Design review of the part shown in the three views and the two pictorial views. Dimensions are in mm from the part's minimum x, y and z. A direction names the side the tool comes from. Round coordinates to 2 decimals unless told otherwise and drop trailing zeros. Order: outer loops, then holes, each group sorted by start corner. A loop starts at its lowest first (then second) coordinate and runs counter-clockwise, first axis right, second up. Notation, with made-up numbers: (89.5, 13.5) - (133.5, 13.5) arc R9 cw to (133.5, 23.5) - close; hole circle Ø4 at (33, 74). An arc over 180 degrees is marked (long way). One line per item, written item: value.
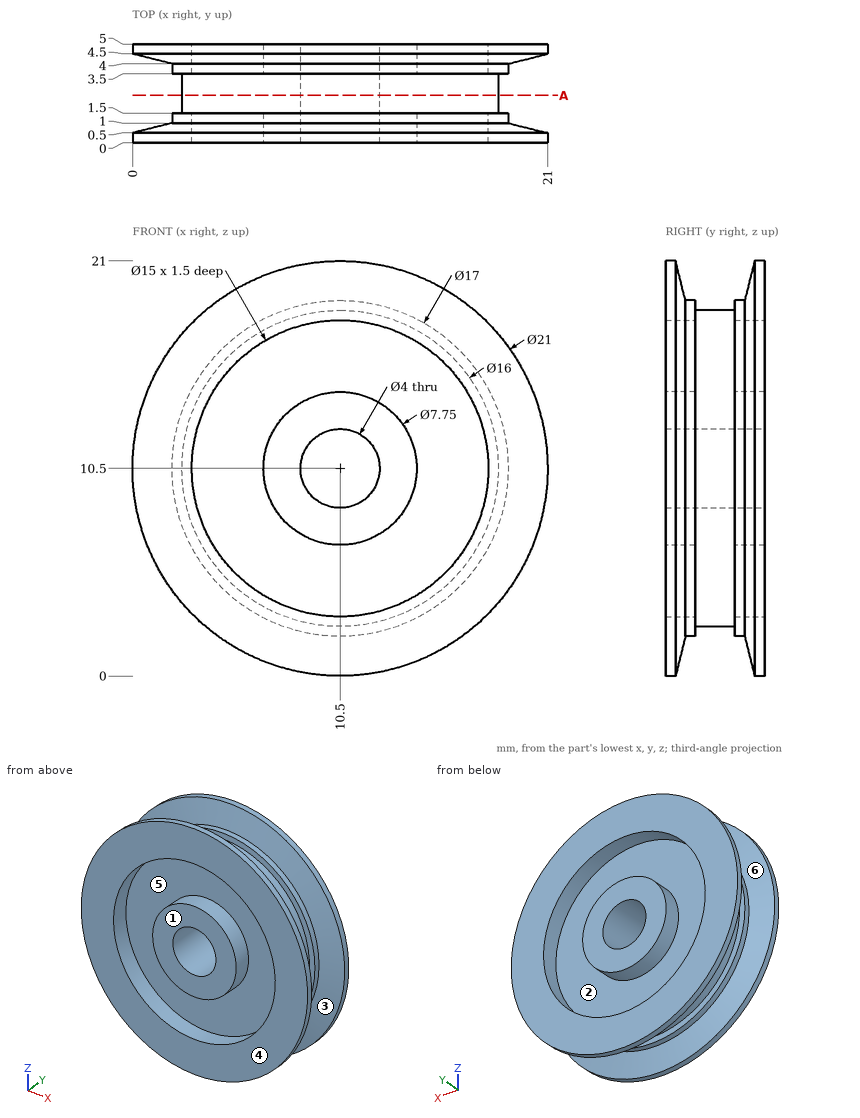
Item 1: Wall thickness on line 1 (X direction, y = 1.1, z = 10.5) (3 decimals); line 2 (X direction, y = 4.55, z = 10.5) (3 decimals); line 3 (X direction, y = 1.7, z = 10.5): over which ranges is each line inside the solid? List them lowest first.
Returned:
line 1: 2 to 3, 6.625 to 8.5, 12.5 to 14.375, 18 to 19
line 2: 0 to 3, 6.625 to 8.5, 12.5 to 14.375, 18 to 21
line 3: 2.5 to 8.5, 12.5 to 18.5
Item 2: Take a section at A-A (y = 2.4). Write out the cut boundary in (x, z), plus the area to 3 significant figures.
Returned:
outline: circle Ø16 at (10.5, 10.5); hole circle Ø4 at (10.5, 10.5)
area: 188 mm^2
Item 3: For P1, Ø12, axis at x = 13, z = 7, coming from the -Y side; P2, Ø1.5, axis at y = 1, z = 3.5, coming from the +X side; P3, Ø1.5, axis at y = 0.5, z = 15.5, coming from the +X side, all flat-tipped, find the tip position at first contact; note any pin that passes through.
Returned:
P1: y = 0
P2: x = 18.79
P3: x = 20.1
Item 4: Machinability: for the marked faces 1, 2 and 3, which of the approach directions +Z, -Z, +X, -X, +Y, -Y give a long, thin tool a straight path to every point of the face, cutting with its end or side? Answer none if there is none.
Returned:
face 1: +Z, -Z, +X, -X, -Y
face 2: +Y
face 3: none
Item 5: The part is to be moulded in two halves that separate along Z. For the marked faces 4, 5 and 6, say which applies: +Z half, -Z half, draft (parallel to the pull), parting line (faces both ways), or undercut.
Returned:
face 4: draft
face 5: undercut
face 6: parting line
